Part print with two shaded views. Sizes in mm from the minimum x, y, z corner. Round coordinates to 2 decimals unless told otherwise and drop trailing zeros. Loops run counter-clockwise (first coordinate to the right, second up) from the corner with the lowest first, then second, coordinate; pieces in that order, holes last.
(1) Flat gauge pins, fed straight in: pin 1 (2.5 mm diameter, centred on x = 114.3, z = 15.24, fed in from -Y); pin 2 (5.5 mm diameter, centred on x = 38.1, z = 15.24, fed in from +Y). Where does each tip first touch, or does it go through?
(2) Probe probe 1 along Z at (x, y) = (38.1, 2.7); probe 2 along Z at (x, y) = (37, 2.5); probe 3 along X at (y, z) = (2.5, 33) (1 decimal). List the from-to ranges inside material, lowest first.
(3) Cut at A-A on z = 15.24. Count the separate pieces of the cut face and the enclosed holes in it.
(4) Cut at D-D on z = 43.5. List the corners of the cut face in (x, y).
(5) Cut at B-B on x = 38.1. List the corners of the cut face in (y, z) (1 decimal).
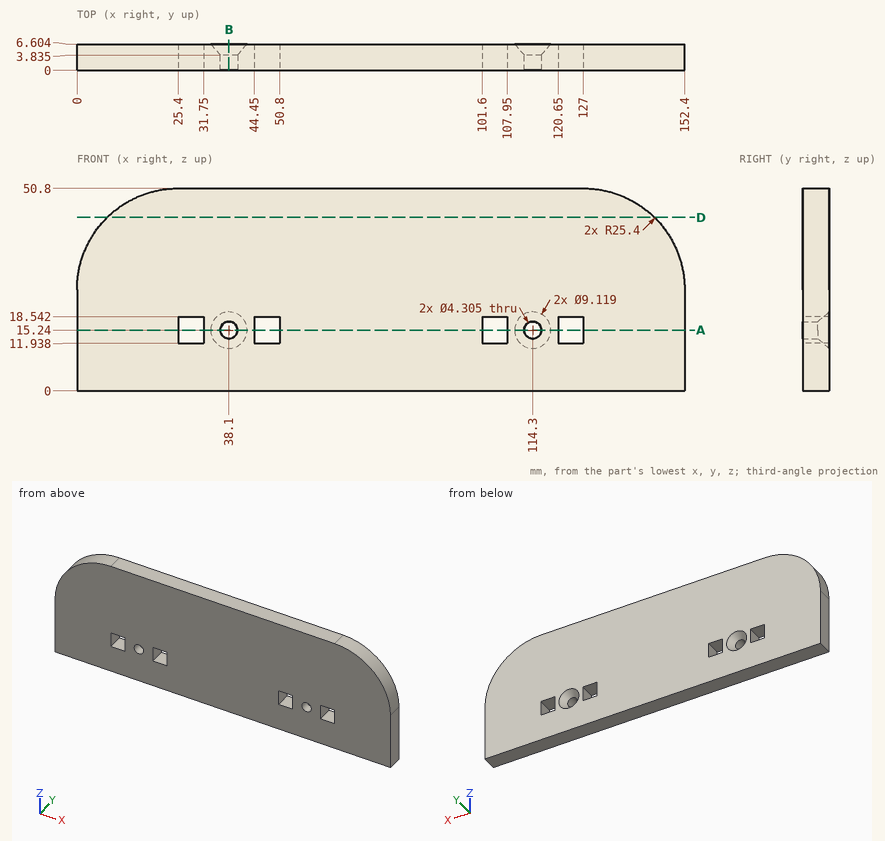
Final values:
1. pin 1: passes through
1. pin 2: stops at y = 4.52
2. probe 1: z = 0 to 13.09, 17.39 to 50.8
2. probe 2: z = 0 to 13.39, 17.09 to 50.8
2. probe 3: x = 1.2 to 151.2
3. separate pieces: 7
3. enclosed holes: 0
4. outline: (7.58, 0) - (144.82, 0) - (144.82, 6.6) - (7.58, 6.6) - close
5. outline: (0, 0) - (6.6, 0) - (6.6, 10.7) - (3.8, 13.1) - (0, 13.1) - close; (0, 17.4) - (3.8, 17.4) - (6.6, 19.8) - (6.6, 50.8) - (0, 50.8) - close
